from build123d import *

# Parameters (mm, degrees)
BOSS_EXTRUDE1_DEPTH = 50.8
SKETCH2_W           = 25.4
SKETCH2_H           = 3.175
BOSS_EXTRUDE2_DEPTH = 304.8
BOSS_EXTRUDE4_DEPTH = 50.8


with BuildPart() as part:
    # Sketch1 → Boss-Extrude1 (new body)
    with BuildSketch(Plane.XY):
        Polygon((-29.786832061, -3.837169287), (-4.386832061, -3.837169287), (30.02261423, 116.162830713), (157.02261423, 116.162830713), (191.432060521, -3.837169287), (216.832060521, -3.837169287), (216.832060521, -7.012169287), (189.039526412, -7.012169287), (154.630080121, 112.987830713), (32.415148339, 112.987830713), (-1.994297952, -7.012169287), (-29.786832061, -7.012169287), align=None)
    extrude(amount=BOSS_EXTRUDE1_DEPTH)

    # Sketch2 → Boss-Extrude2 (add)
    with BuildSketch(Plane.XY.offset(50.8)):
        with Locations((68.12261423, 114.575330713)):
            Rectangle(SKETCH2_W, SKETCH2_H)
        with Locations((118.92261423, 114.575330713)):
            Rectangle(SKETCH2_W, SKETCH2_H)
    extrude(amount=BOSS_EXTRUDE2_DEPTH)

    # Sketch4 → Boss-Extrude4 (add)
    with BuildSketch(Plane.XY.offset(355.6)):
        Polygon((30.02261423, 116.162830713), (157.02261423, 116.162830713), (191.432060521, -3.837169287), (216.832060521, -3.837169287), (216.832060521, -7.012169287), (189.039526412, -7.012169287), (154.630080121, 112.987830713), (32.415148339, 112.987830713), (-1.994297952, -7.012169287), (-29.786832061, -7.012169287), (-29.786832061, -3.837169287), (-4.386832061, -3.837169287), align=None)
    extrude(amount=BOSS_EXTRUDE4_DEPTH)


solid = part.part
Input: part model. Units: mm. Frame: model coordinates. A direction names the side the tool comes from. Coordinates: 2 decimals unless noted, no trailing zeros. Order: outer loops, then holes, each group sorted by start corner. A loop starts at its lowest first (then second) coordinate and runs counter-clockwise, first axis right, second up.
1. Draft query along X for faces 1 (the flat face through (203, -7.012, 25)), 2 (the flat face through (12.577, 55.323, 25.044)), 3 (the flat face through (173.986, 57.003, 25.044)), 4 (the flat face through (15.45, 53.83, 25.04)). Return one class per face: +X half, -X half, draft (parallel to the pull), parting line (faces both ways), or undercut.
Checked values:
face 1: draft
face 2: -X half
face 3: +X half
face 4: undercut
2. Cut plane B-B, the plane z = 104.5. Return loops of the section in (x, y).
Checked values:
outline: (55.42, 112.99) - (80.82, 112.99) - (80.82, 116.16) - (55.42, 116.16) - close; (106.22, 112.99) - (131.62, 112.99) - (131.62, 116.16) - (106.22, 116.16) - close
3. Cut plane A-A, the plane x = 37. Return loops of the section in (y, z).
Checked values:
outline: (112.99, 0) - (116.16, 0) - (116.16, 50.8) - (112.99, 50.8) - close; (112.99, 355.6) - (116.16, 355.6) - (116.16, 406.4) - (112.99, 406.4) - close
4. Ray query, line 1 along Y through (x, z) = (123, 291); line 2 along Y through (x, z) = (198, 41); line 3 along X through (y, z) = (48, 377). Return the intervals inside material, ascending.
Checked values:
line 1: y = 112.99 to 116.16
line 2: y = -7.01 to -3.84
line 3: x = 10.48 to 13.78, 173.27 to 176.57
5. Access query for faces 5 (the flat face through (15.45, 53.83, 380.64)), 6 (the flat face through (13, 55, 355.6)), 7 (the flat face through (-17, -3.837, 381)). Directions: +Z, -Z, +X, -X, +Y, -Y. A direction counts if a zero-diameter tool reaches every point of the face in a straight line with its end or side. Return the directions, or none.
Checked values:
face 5: +Z, -Z, -Y
face 6: -X, +Y, -Y
face 7: +Z, -Z, -X, +Y
6. Contact query for flat-ended pins moving along their axis: P1, Ø20.5, axis at x = 209, z = 22, coming from the +Y side; P2, Ø1, axis at x = 181.5, y = 37.5, coming from the +Z side; P3, Ø5, axis at x = 53, z = 278.5, coming from the +Y side; P4, Ø1, axis at y = 114.5, z = 234.5, coming from the -X side. Output: stop coordinate, or through.
Checked values:
P1: stops at y = -3.84
P2: passes through
P3: stops at y = 116.16
P4: stops at x = 55.42
7. Cut plane C-C, the plane y = 51.5. Return loops of the section in (x, z).
Checked values:
outline: (11.48, 0) - (14.78, 0) - (14.78, 50.8) - (11.48, 50.8) - close; (11.48, 355.6) - (14.78, 355.6) - (14.78, 406.4) - (11.48, 406.4) - close; (172.26, 0) - (175.56, 0) - (175.56, 50.8) - (172.26, 50.8) - close; (172.26, 355.6) - (175.56, 355.6) - (175.56, 406.4) - (172.26, 406.4) - close
